from build123d import *

# Parameters (mm, degrees)
SKETCH1_R           = 7.8
BOSS_EXTRUDE1_DEPTH = 31
CHAMFER1_SIZE       = 1
CHAMFER2_SIZE       = 1
CHAMFER3_SIZE       = 1
CHAMFER4_SIZE       = 1
SKETCH2_R           = 2
CUT_EXTRUDE1_DEPTH  = 18
SKETCH3_R           = 8.8
CUT_EXTRUDE2_DEPTH  = 3.5
CUT_EXTRUDE3_START  = -3.5
SKETCH4_R           = 8.8
CUT_EXTRUDE3_DEPTH  = 3.5
BOSS_EXTRUDE2_START = -2.5
SKETCH5_R           = 8.8
SKETCH5_R_2         = 7.8
BOSS_EXTRUDE2_DEPTH = 2.5
SKETCH6_R           = 8.8
SKETCH6_R_2         = 7.8
BOSS_EXTRUDE3_DEPTH = 2.5


with BuildPart() as part:
    # Sketch1 → Boss-Extrude1 (new body)
    with BuildSketch(Plane.XY):
        Polygon((-6, -7.931107296), (6, -7.931107296), (6, -8.431107296), (17, -8.431107296), (17, -0.931107296), (16.5, -0.931107296), (16.5, 9.568892704), (8, 9.568892704), (4, 13.568892704), (-4, 13.568892704), (-8, 9.568892704), (-16.5, 9.568892704), (-16.5, -0.931107296), (-17, -0.931107296), (-17, -8.431107296), (-6, -8.431107296), align=None)
        with Locations((0, 2.568892704)):
            Circle(SKETCH1_R, mode=Mode.SUBTRACT)
    extrude(amount=BOSS_EXTRUDE1_DEPTH)

    # Chamfer1
    chamfer1_edges = [part.edges().sort_by_distance(p)[0] for p in [
        (-16.5, 9.568892704, 15.5),
        (16.5, 9.568892704, 15.5),
    ]]
    chamfer(chamfer1_edges, length=CHAMFER1_SIZE)

    # Chamfer2
    # the kernel refuses this chamfer: 1 mm, written as the material it takes off along each edge
    with BuildSketch(Plane(origin=(-17, -0.931107296, -2.571682988), x_dir=(-0.02749587661058563, -0.9996219169112968, 0), z_dir=(0, 0, 1))) as chamfer2_piece_1_section:
        Polygon((CHAMFER2_SIZE * 0.999621916911, CHAMFER2_SIZE * 0.0274958766106), (-CHAMFER2_SIZE * 0.0274958766106, CHAMFER2_SIZE * 0.999621916911), (0, 0), align=None)
    chamfer2_piece_1 = extrude(amount=36.143365976, mode=Mode.PRIVATE)
    chamfer2_piece_1 = split(chamfer2_piece_1, bisect_by=Plane(origin=(-16.5, -1.32450838, 15.5), z_dir=(-1, 0, 0)), keep=Keep.TOP, mode=Mode.PRIVATE)
    add(chamfer2_piece_1, mode=Mode.SUBTRACT)
    with BuildSketch(Plane(origin=(17, -0.931107296, -2.571682988), x_dir=(-0.9996219169112968, 0.027495876610586403, 0), z_dir=(0, 0, 1))) as chamfer2_piece_2_section:
        Polygon((CHAMFER2_SIZE * 0.999621916911, CHAMFER2_SIZE * 0.0274958766106), (-CHAMFER2_SIZE * 0.0274958766106, CHAMFER2_SIZE * 0.999621916911), (0, 0), align=None)
    chamfer2_piece_2 = extrude(amount=36.143365976, mode=Mode.PRIVATE)
    chamfer2_piece_2 = split(chamfer2_piece_2, bisect_by=Plane(origin=(16.5, -1.32450838, 15.5), z_dir=(1, 0, 0)), keep=Keep.TOP, mode=Mode.PRIVATE)
    add(chamfer2_piece_2, mode=Mode.SUBTRACT)

    # Chamfer3
    chamfer3_edges = [part.edges().sort_by_distance(p)[0] for p in [
        (-17, -8.431107296, 15.5),
        (17, -8.431107296, 15.5),
    ]]
    chamfer(chamfer3_edges, length=CHAMFER3_SIZE)

    # Chamfer4
    # the kernel refuses this chamfer: 1 mm, written as the material it takes off along each edge
    with BuildSketch(Plane(origin=(-6, -8.431107296, -2.571682988), x_dir=(-0.9996219169112968, -0.027495876610585623, 0), z_dir=(0, 0, 1))) as chamfer4_piece_1_section:
        Polygon((CHAMFER4_SIZE * 0.999621916911, -CHAMFER4_SIZE * 0.0274958766106), (-CHAMFER4_SIZE * 0.0274958766106, -CHAMFER4_SIZE * 0.999621916911), (0, 0), align=None)
    chamfer4_piece_1 = extrude(amount=36.143365976, mode=Mode.PRIVATE)
    chamfer4_piece_1 = split(chamfer4_piece_1, bisect_by=Plane(origin=(-6.393401084, -7.931107296, 15.5), z_dir=(0, -1, 0)), keep=Keep.TOP, mode=Mode.PRIVATE)
    add(chamfer4_piece_1, mode=Mode.SUBTRACT)
    with BuildSketch(Plane(origin=(6, -8.431107296, -2.571682988), x_dir=(-0.027495876610586487, 0.9996219169112968, 0), z_dir=(0, 0, 1))) as chamfer4_piece_2_section:
        Polygon((CHAMFER4_SIZE * 0.999621916911, -CHAMFER4_SIZE * 0.0274958766106), (-CHAMFER4_SIZE * 0.0274958766106, -CHAMFER4_SIZE * 0.999621916911), (0, 0), align=None)
    chamfer4_piece_2 = extrude(amount=36.143365976, mode=Mode.PRIVATE)
    chamfer4_piece_2 = split(chamfer4_piece_2, bisect_by=Plane(origin=(6.393401084, -7.931107296, 15.5), z_dir=(0, -1, 0)), keep=Keep.TOP, mode=Mode.PRIVATE)
    add(chamfer4_piece_2, mode=Mode.SUBTRACT)

    # Sketch2 → Cut-Extrude1 (cut)
    with BuildSketch(Plane.XZ.offset(8.431107296)):
        with Locations(Location((-12, 6.5, 0), (0, 0, 270))):
            Circle(SKETCH2_R)
        with Locations(Location((-12, 24.5, 0), (0, 0, 270))):
            Circle(SKETCH2_R)
        with Locations(Location((12, 6.5, 0), (0, 0, 270))):
            Circle(SKETCH2_R)
        with Locations(Location((12, 24.5, 0), (0, 0, 270))):
            Circle(SKETCH2_R)
    extrude(amount=-CUT_EXTRUDE1_DEPTH, mode=Mode.SUBTRACT)

    # Sketch3 → Cut-Extrude2 (cut)
    with BuildSketch(Plane.XY.offset(31)):
        with Locations((0, 2.568892704)):
            Circle(SKETCH3_R)
    extrude(amount=-CUT_EXTRUDE2_DEPTH, mode=Mode.SUBTRACT)

    # Sketch4 → Cut-Extrude3 (cut)
    with BuildSketch(Plane(origin=(0, 0, 0), x_dir=(-1, 0, 0), z_dir=(0, 0, -1)).offset(CUT_EXTRUDE3_START)):
        with Locations(Location((0, 2.568892704, 0), (0, 0, 180))):
            Circle(SKETCH4_R)
    extrude(amount=CUT_EXTRUDE3_DEPTH, mode=Mode.SUBTRACT)

    # Sketch5 → Boss-Extrude2 (add)
    with BuildSketch(Plane(origin=(0, 0, 0), x_dir=(-1, 0, 0), z_dir=(0, 0, -1)).offset(BOSS_EXTRUDE2_START)):
        with Locations((0, 2.568892704)):
            Circle(SKETCH5_R)
        with Locations((0, 2.568892704)):
            Circle(SKETCH5_R_2, mode=Mode.SUBTRACT)
    extrude(amount=BOSS_EXTRUDE2_DEPTH)

    # Sketch6 → Boss-Extrude3 (add)
    with BuildSketch(Plane.XY.offset(31)):
        with Locations((0, 2.568892704)):
            Circle(SKETCH6_R)
        with Locations(Location((0, 2.568892704, 0), (0, 0, 180))):
            Circle(SKETCH6_R_2, mode=Mode.SUBTRACT)
    extrude(amount=-BOSS_EXTRUDE3_DEPTH)


solid = part.part
The model under review builds one solid part; all positions refer to its coordinate system, in mm. A direction names the side the tool comes from. Coordinates: 2 decimals unless noted, no trailing zeros. Write each loop counter-clockwise with the first axis right and the second up, starting at its lowest first coordinate (ties: lowest second). Pieces come first, ordered by that corner, then holes. Notation, with made-up numbers: M 73.25,52.25 L 121.25,52.25 A27 cw 121.25,73.25 Z; hole C 55.25,83.25 d7. An arc over 180 degrees is marked long. Put each result on its own line as item: value.
1) Add section A-A on y = -4. Give the boundary of the cut face in (x, z), then the cut area to 3 significant figures.
Computed:
outline: M -17,0 L -4.21,0 L -4.21,2.5 L -5.86,2.5 L -5.86,3.5 L -4.21,3.5 L -4.21,27.5 L -5.86,27.5 L -5.86,28.5 L -4.21,28.5 L -4.21,31 L -17,31 Z; M 4.21,0 L 17,0 L 17,31 L 4.21,31 L 4.21,28.5 L 5.86,28.5 L 5.86,27.5 L 4.21,27.5 L 4.21,3.5 L 5.86,3.5 L 5.86,2.5 L 4.21,2.5 Z; hole C -12,6.5 d4; hole C -12,24.5 d4; hole C 12,6.5 d4; hole C 12,24.5 d4
area: 736 mm2
2) Clearance check with flat-ended pins moving along their axes: pin 1 Ø2 at (x, z) = (-3.5, 6) entering from -Y; pin 2 Ø5 at (y, z) = (3.5, 17) entering from +X; pin 3 Ø3 at (x, z) = (7, 27) entering from +Y. State where each tip first meets the part, or that it passes through.
Computed:
pin 1: stops at y = -7.93
pin 2: stops at x = 16.5
pin 3: stops at y = 12.07
3) Draft analysis for pull direction Y (two halves, no side actions). For faces 1 (the flat face through (12, 9.569, 15)), 2 (the cylindrical face through (-1.1, 11.3, 28)), 3 (the flat face through (16.5, 3, 15)), state which applies: released by +Y, released by -Y, zero draft, split by the parting line, or undercut.
Computed:
face 1: released by +Y
face 2: undercut
face 3: zero draft
4) Add section C-C on x = 0. Give the boundary of the cut face in (y, z), then the cut area to 3 significant figures.
Computed:
outline: M -7.93,0 L -5.23,0 L -5.23,2.5 L -6.23,2.5 L -6.23,3.5 L -5.23,3.5 L -5.23,27.5 L -6.23,27.5 L -6.23,28.5 L -5.23,28.5 L -5.23,31 L -7.93,31 Z; M 10.37,0 L 13.57,0 L 13.57,31 L 10.37,31 L 10.37,28.5 L 11.37,28.5 L 11.37,27.5 L 10.37,27.5 L 10.37,3.5 L 11.37,3.5 L 11.37,2.5 L 10.37,2.5 Z
area: 179 mm2
5) Add section D-D on x = 12. Give the boundary of the cut face in (y, z), then the cut area to 3 significant figures.
Computed:
outline: M -8.43,0 L 9.57,0 L 9.57,4.5 L -8.43,4.5 Z; M -8.43,8.5 L 9.57,8.5 L 9.57,22.5 L -8.43,22.5 Z; M -8.43,26.5 L 9.57,26.5 L 9.57,31 L -8.43,31 Z
area: 414 mm2
6) Wall thickness on probe 1 along Z at (x, y) = (-6.5, 7); probe 2 along X at (y, z) = (-7.5, 6.5); probe 3 along X at (y, z) = (8.5, 8): over which ranges is each line inside the solid? List them lowest first. Write a range as [from, to].
Computed:
probe 1: z = [0, 2.5], [3.5, 27.5], [28.5, 31]
probe 2: x = [-16.93, -14], [-10, 10], [14, 16.93]
probe 3: x = [-16.5, -13.32], [-10.68, -5.07], [5.07, 10.68], [13.32, 16.5]
7) Add section B-B on z = 6.5. State how many separate pieces and enclosed holes the cut face has, then the cut area to 3 significant figures.
Computed:
separate pieces: 3
enclosed holes: 1
area: 305 mm2
8) For faces 4 (the cylindrical face through (-6.19, -2.18, 15.33)), 5 (the flat face through (-3, -5, 28.5)), list the 3-axis set-ups (+Z, -Z, +X, -X, +Y, -Y) from which the entire face can be reached by the end or side of a thin tool; tool diameter is ignored.
Computed:
face 4: +Z, -Z
face 5: none
